Here's how the part is built. I have some questions about the finished solid (model axes, mm). Round coordinates to 2 decimals unless told otherwise and drop trailing zeros. Write each loop counter-clockwise with the first axis right and the second up, starting at its lowest first coordinate (ties: lowest second). Pieces come first, ordered by that corner, then holes. Notation, with made-up numbers: (30, -21) -> (89, -21) arc R20 cw to (89, 1) -> close; hole circle Ø5 at (31.5, 86). An arc over 180 degrees is marked (long way). Answer as CSV lines item,"result".
from build123d import *

# Parameters (mm, degrees)
SKETCH1_W           = 158.75
SKETCH1_H           = 304.8
SKETCH1_R           = 57.5
SKETCH1_W_2         = 130.175
SKETCH1_H_2         = 30.1625
SKETCH1_W_3         = 127
SKETCH1_H_3         = 12.7
BOSS_EXTRUDE1_DEPTH = 3.175


with BuildPart() as part:
    # Sketch1 → Boss-Extrude1 (new body)
    with BuildSketch(Plane(origin=(0, 0, 0), x_dir=(1, 0, 0), z_dir=(0, 1, 0))):
        with Locations((79.375, 152.4)):
            Rectangle(SKETCH1_W, SKETCH1_H)
        with Locations(Location((79.375, 209.2, 0), (0, 0, 270))):
            Circle(SKETCH1_R, mode=Mode.SUBTRACT)
        with Locations((79.375, 133.432370025)):
            Rectangle(SKETCH1_W_2, SKETCH1_H_2, mode=Mode.SUBTRACT)
        with Locations((79.375, 104.734192112)):
            Rectangle(SKETCH1_W_3, SKETCH1_H_3, mode=Mode.SUBTRACT)
    extrude(amount=BOSS_EXTRUDE1_DEPTH)


solid = part.part
Item 1: Suppose I cut it at D-D, the plane y = 1.35. State how many separate pieces and enclosed holes the cut face has, then the cut area to 3 significant figures.
Results found:
separate pieces,"1"
enclosed holes,"3"
area,"32,500 mm²"
Item 2: Suppose I cut it at C-C, the plane x = 36. List the corners of the cut face in (y, z) for me (3 decimals), then the cut area to 3 significant figures.
Results found:
outline,"(0, -304.8) -> (3.175, -304.8) -> (3.175, -246.947) -> (0, -246.947) -> close; (0, -171.453) -> (3.175, -171.453) -> (3.175, -148.514) -> (0, -148.514) -> close; (0, -118.351) -> (3.175, -118.351) -> (3.175, -111.084) -> (0, -111.084) -> close; (0, -98.384) -> (3.175, -98.384) -> (3.175, 0) -> (0, 0) -> close"
area,"592 mm²"
Item 3: I need wall thicknesses on L1, parallel to X at y = 2.3, z = -101.5 (3 decimals); L2, parallel to Z at x = 45.5, y = 1.5; L3, parallel to Z at x = 118, y = 1.55. Which ranges of each line are inside material? Lowest first, please.
Results found:
L1,"x = 0 to 15.875, 142.875 to 158.75"
L2,"z = -304.8 to -255.66, -162.74 to -148.51, -118.35 to -111.08, -98.38 to 0"
L3,"z = -304.8 to -251.8, -166.6 to -148.51, -118.35 to -111.08, -98.38 to 0"
Item 4: If we mould it in two halves opening along Z, with no side actions, what happens to faces 1 (the cylindrical face through (96.646, 1.565, -154.355)), 2 (the flat face through (60.6, 3.175, -154.5))? For each: pulls with the +Z half, pulls with the -Z half, needs draft (parallel to the pull), parting line crosses it, or undercut.
Results found:
face 1,"undercut"
face 2,"needs draft"
Item 5: Suppose I cut it at B-B, the plane z = -209.2. List the corners of the cut face in (x, y) for me (3 decimals), then the cut area to 3 significant figures.
Results found:
outline,"(0, 0) -> (21.875, 0) -> (21.875, 3.175) -> (0, 3.175) -> close; (136.875, 0) -> (158.75, 0) -> (158.75, 3.175) -> (136.875, 3.175) -> close"
area,"139 mm²"
Item 6: Will this pin go through, and if not, where does the flat tip stop? pin 1 (1.6 mm diameter, centred on y = 2, z = -106.5, fed in from -X).
Results found:
pin 1,"stops at x = 0"
